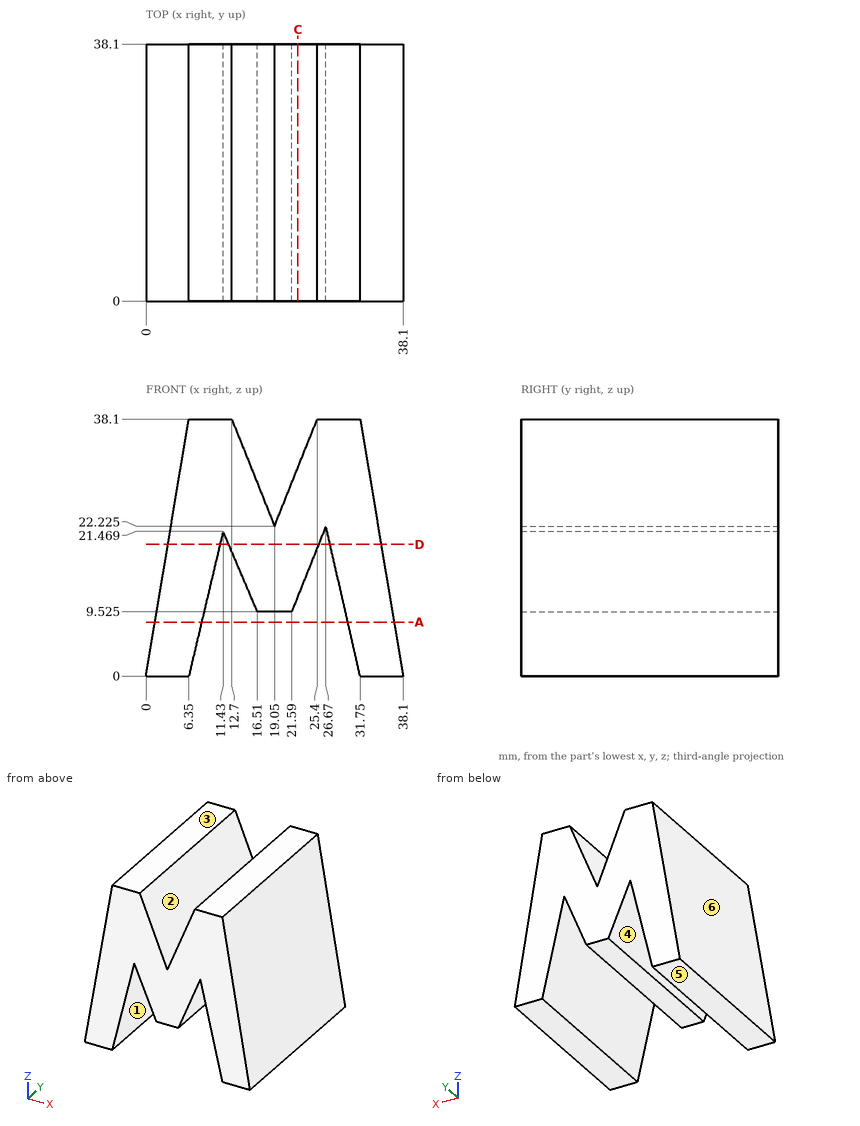
Can you work these out from the drawing? Everything is in mm from the part's minimum corner. A direction names the side the tool comes from. Give positions to 0.01 mm unless a question says otherwise; leave off trailing zeros. Loops run counter-clockwise (first coordinate to the right, second up) from the corner with the lowest first, then second, coordinate; pieces in that order, holes last. Notation, with made-up numbers: M -26,68.25 L 9,68.25 A23 cw 9,84.25 Z; hole C 71,84.25 d3. An arc over 180 degrees is marked long. Put each result on its own line as item: value. Start each with the question number.
(1) I want a section at D-D on z = 19.5. Please give me the cut outline in (x, y), then the cut area to 3 significant figures.
(2) For the marked faces 1, 2 and 3, which set-ups out of +Z, -Z, +X, -X, +Y, -Y let a thin tool reach every point of the face, with its end or its side?
(3) I want a section at C-C on x = 22.5. Please give me the cut outline in (y, z).
(4) I need wall thicknesses on line 1 along X through (y, z) = (10, 23) (1 decimal); line 2 along X through (y, z) = (6, 28) (1 decimal); line 3 along X through (y, z) = (33, 18) (1 decimal). Which ranges of each line are inside material? Lowest first, please. Write a range as [from, to].
(5) If we mould it in two halves opening along X, with no side actions, what happens to the marked faces 4, 5 and 6? For each: +X half, -X half, draft (parallel to the pull), parting line (faces both ways), or undercut.
(6) Will these pins go through, and if not, where does the flat tip stop? pin 1 Ø1.5 at (y, z) = (23, 5.5) entering from +X; pin 2 Ø6 at (y, z) = (16, 23.5) entering from -X; pin 3 Ø3 at (y, z) = (19, 27) entering from +X.
(7) I want a section at A-A on z = 8. Please give me the cut outline in (x, y), then the cut area to 3 significant figures.
Answer block:
1. outline: M 3.25,0 L 10.96,0 L 10.96,38.1 L 3.25,38.1 Z; M 12.27,0 L 25.58,0 L 25.58,38.1 L 12.27,38.1 Z; M 27.29,0 L 34.85,0 L 34.85,38.1 L 27.29,38.1 Z
1. area: 1,090 mm^2
2. face 1: -Z, +Y, -Y
2. face 2: +Z, +Y, -Y
2. face 3: +Z, +X, -X, +Y, -Y
3. outline: M 0,11.8 L 38.1,11.8 L 38.1,30.85 L 0,30.85 Z
4. line 1: [3.8, 18.7], [19.4, 34.3]
4. line 2: [4.7, 16.7], [21.4, 33.4]
4. line 3: [3, 10.6], [12.9, 25], [27.6, 35.1]
5. face 4: undercut
5. face 5: draft
5. face 6: -X half
6. pin 1: x = 37.31
6. pin 2: x = 3.42
6. pin 3: x = 33.85
7. outline: M 1.33,0 L 8.24,0 L 8.24,38.1 L 1.33,38.1 Z; M 29.92,0 L 36.77,0 L 36.77,38.1 L 29.92,38.1 Z
7. area: 524 mm^2
